Could you check a few things on this drawing? It's one solid part, dimensions in mm from its lowest x, y, z. A direction names the side the tool comes from. Round coordinates to 2 decimals unless told otherwise and drop trailing zeros. Loops run counter-clockwise (first coordinate to the right, second up) from the corner with the lowest first, then second, coordinate; pieces in that order, holes last. Notation, with made-up numbers: M 71.25,-15 L 92.25,-15 A27 cw 92.25,11 Z; hole C -30,-12.75 d5. An arc over 180 degrees is marked long. Return JSON: item names as keys, results as strings.
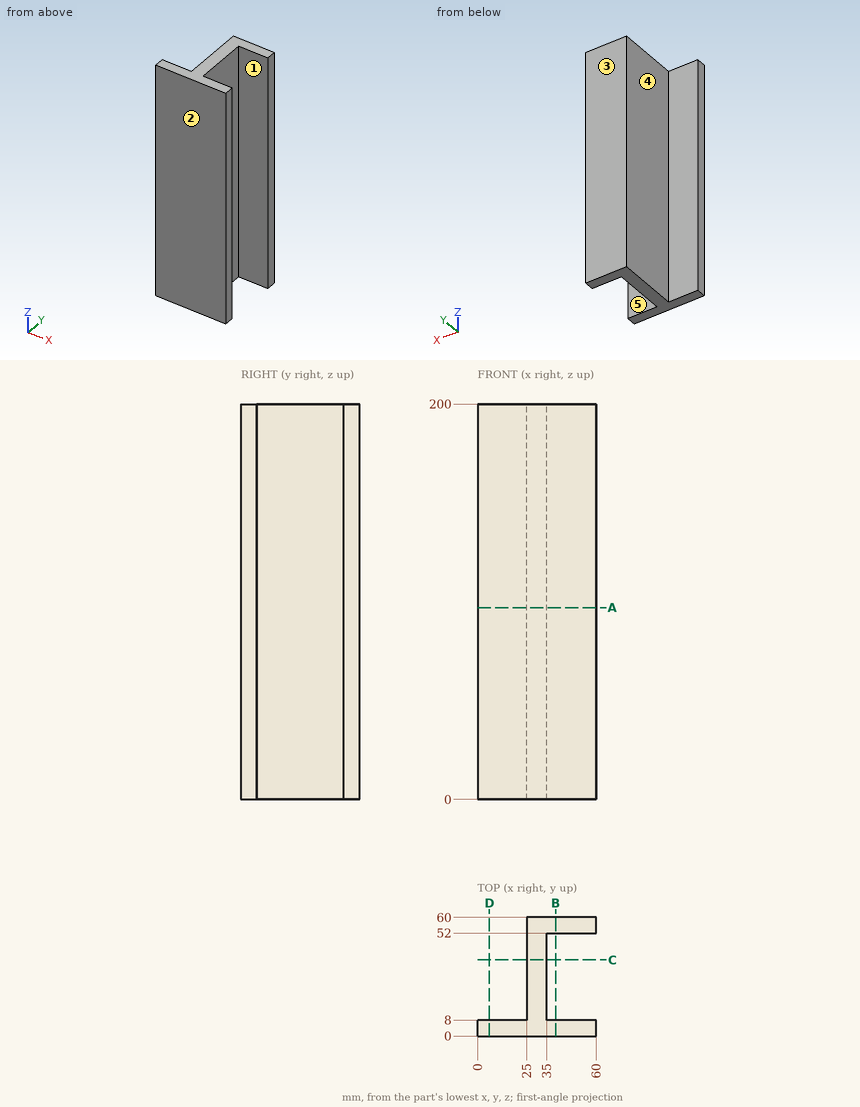
Q1. On a 3-axis mill with a long thin cutter (end or side, diameter ignored), from which of +Z, -Z, +X, -X, +Y, -Y can I reach the whole of each face in a straight line? I mean the marked faces 4 and 5. Say none if no direction works.
Results:
{"face 4": "+Z, -Z, -X, +Y", "face 5": "+Z, -Z, +X"}
Q2. Suppose I cut it at D-D, the plane x = 6. Please give me the cut outline in (y, z), plus the area to 3 significant figures.
Results:
{"outline": "M 0,0 L 8,0 L 8,200 L 0,200 Z", "area": "1,600 mm2"}
Q3. I'm going to push flat-ended pins straight in: pin 1 Ø12.5 at (x, z) = (49.5, 133) entering from -Y; pin 2 Ø12 at (x, y) = (43, 24) entering from +Z; pin 3 Ø5 at (y, z) = (35, 145) entering from -X; pin 4 Ø3 at (x, z) = (11.5, 135.5) entering from +Y. Where does each tip first touch, or does it pass through?
Results:
{"pin 1": "stops at y = 0", "pin 2": "passes through", "pin 3": "stops at x = 25", "pin 4": "stops at y = 8"}
Q4. If I drill on line 1 along Y through (x, z) = (48.5, 143); line 2 along Y through (x, z) = (9.5, 126.5); line 3 along X through (y, z) = (38.5, 101), over which ranges is the centre line in solid material (lowest first)?
Results:
{"line 1": "y = 0 to 8, 52 to 60", "line 2": "y = 0 to 8", "line 3": "x = 25 to 35"}
Q5. Thinking about a two-plate mould opening in Y: for the marked faces 1, 2 and 3, which applies, pulls with the +Y half, pulls with the -Y half, needs draft (parallel to the pull), parting line crosses it, or undercut?
Results:
{"face 1": "undercut", "face 2": "pulls with the -Y half", "face 3": "pulls with the +Y half"}
Q6. Suppose I cut it at B-B, the plane x = 39.5. Please give me the cut outline in (y, z), plus the area to 3 significant figures.
Results:
{"outline": "M 0,0 L 8,0 L 8,200 L 0,200 Z; M 52,0 L 60,0 L 60,200 L 52,200 Z", "area": "3,200 mm2"}
Q7. Suppose I cut it at A-A, the plane z = 97. Please give me the cut outline in (x, y), plus the area to 3 significant figures.
Results:
{"outline": "M 0,0 L 60,0 L 60,8 L 35,8 L 35,52 L 60,52 L 60,60 L 25,60 L 25,8 L 0,8 Z", "area": "1,200 mm2"}
Q8. Suppose I cut it at C-C, the plane y = 38.5. Please give me the cut outline in (x, z).
Results:
{"outline": "M 25,0 L 35,0 L 35,200 L 25,200 Z"}
